The model under review builds one solid part; all positions refer to its coordinate system, in mm. Face numbers are marked on the shaded views. A direction names the side the tool comes from. Round coordinates to 2 decimals unless told otherwise and drop trailing zeros. Loops run counter-clockwise (first coordinate to the right, second up) from the corner with the lowest first, then second, coordinate; pieces in that order, holes last. Notation, with made-up numbers: M 9,-22.5 L 36,-22.5 A31 cw 36,2.5 Z; hole C 14.25,55 d9. An arc over 180 degrees is marked long. Answer in a Markdown table with one row per item. Add a question column.
from build123d import *

# Parameters (mm, degrees)
SCHIZZO1_W                   = 41
SCHIZZO1_H                   = 41
ESTRUSIONE_ESTRUSIONE1_DEPTH = 1.5
SCHIZZO5_W                   = 4.5
SCHIZZO5_H                   = 4.5
ESTRUSIONE_ESTRUSIONE2_DEPTH = 6.97
SCHIZZO6_W                   = 4.5
SCHIZZO6_H                   = 4.5
ESTRUSIONE_ESTRUSIONE3_DEPTH = 6.97
SCHIZZO7_W                   = 4.5
SCHIZZO7_H                   = 4.5
ESTRUSIONE_ESTRUSIONE4_DEPTH = 6.97
SCHIZZO8_W                   = 4.5
SCHIZZO8_H                   = 4.5
ESTRUSIONE_ESTRUSIONE5_DEPTH = 6.97
SCHIZZO9_W                   = 1
SCHIZZO9_H                   = 41
ESTRUSIONE_ESTRUSIONE6_DEPTH = 12
SCHIZZO10_W                  = 26
SCHIZZO10_H                  = 1
ESTRUSIONE_ESTRUSIONE7_DEPTH = 12
SCHIZZO11_R                  = 0.4
TAGLIO_ESTRUSIONE1_DEPTH     = 10
SCHIZZO12_R                  = 0.4
TAGLIO_ESTRUSIONE2_DEPTH     = 10


with BuildPart() as part:
    # Schizzo1 → Estrusione-Estrusione1 (new body)
    with BuildSketch(Plane.XY):
        with Locations((20.5, 20.5)):
            Rectangle(SCHIZZO1_W, SCHIZZO1_H)
    extrude(amount=ESTRUSIONE_ESTRUSIONE1_DEPTH)

    # Schizzo5 → Estrusione-Estrusione2 (add)
    with BuildSketch(Plane.XY.offset(1.5)):
        with Locations((2.25, 2.25)):
            Rectangle(SCHIZZO5_W, SCHIZZO5_H)
    extrude(amount=ESTRUSIONE_ESTRUSIONE2_DEPTH)

    # Schizzo6 → Estrusione-Estrusione3 (add)
    with BuildSketch(Plane.XY.offset(1.5)):
        with Locations((38.75, 2.25)):
            Rectangle(SCHIZZO6_W, SCHIZZO6_H)
    extrude(amount=ESTRUSIONE_ESTRUSIONE3_DEPTH)

    # Schizzo7 → Estrusione-Estrusione4 (add)
    with BuildSketch(Plane.XY.offset(1.5)):
        with Locations((2.25, 38.75)):
            Rectangle(SCHIZZO7_W, SCHIZZO7_H)
    extrude(amount=ESTRUSIONE_ESTRUSIONE4_DEPTH)

    # Schizzo8 → Estrusione-Estrusione5 (add)
    with BuildSketch(Plane.XY.offset(1.5)):
        with Locations((38.75, 38.75)):
            Rectangle(SCHIZZO8_W, SCHIZZO8_H)
    extrude(amount=ESTRUSIONE_ESTRUSIONE5_DEPTH)

    # Schizzo9 → Estrusione-Estrusione6 (add)
    with BuildSketch(Plane(origin=(0, 0, 0), x_dir=(-1, 0, 0), z_dir=(0, 0, -1))):
        with Locations((-40.5, 20.5)):
            Rectangle(SCHIZZO9_W, SCHIZZO9_H)
    extrude(amount=ESTRUSIONE_ESTRUSIONE6_DEPTH)

    # Schizzo10 → Estrusione-Estrusione7 (add)
    with BuildSketch(Plane(origin=(0, 0, 0), x_dir=(-1, 0, 0), z_dir=(0, 0, -1))):
        with Locations((-13, 40.5)):
            Rectangle(SCHIZZO10_W, SCHIZZO10_H)
    extrude(amount=ESTRUSIONE_ESTRUSIONE7_DEPTH)

    # Schizzo11 → Taglio-Estrusione1 (cut)
    with BuildSketch(Plane.XY.offset(8.47)):
        with Locations((32.781075858, 214.49933813)):
            Circle(SCHIZZO11_R)
    extrude(amount=-TAGLIO_ESTRUSIONE1_DEPTH, mode=Mode.SUBTRACT)

    # Schizzo12 → Taglio-Estrusione2 (cut)
    with BuildSketch(Plane.XY.offset(8.47)):
        with Locations((-3.518924142, 178.29933813)):
            Circle(SCHIZZO12_R)
    extrude(amount=-TAGLIO_ESTRUSIONE2_DEPTH, mode=Mode.SUBTRACT)


solid = part.part
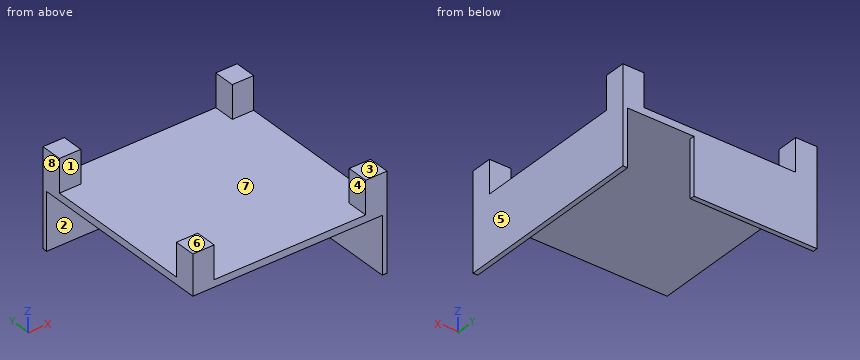
1. Take a section at A-A, the plane z = -1.75. State the section outline as (x, y) points.
2. To check wall thickness, follow probe 1 along Z at (x, y) = (20, 39.5); probe 2 along Y at (x, z) = (6, -10). State the ranges of each line that lie inside material, in increasing order.
3. For pin 1 Ø3 at (x, y) = (9.5, 26) entering from -Z; pin 2 Ø5 at (y, z) = (3.5, 6.5) entering from -X; pin 3 Ø12 at (x, y) = (19.5, 14) entering from +Z; pin 4 Ø10 at (y, z) = (31, -9) entering from -X, all flat-tipped, find the tip position at first contact; note any pin that passes through.
4. Machinability: for the marked faces 1, 2, 3 and 4, which of the approach directions +Z, -Z, +X, -X, +Y, -Y give a long, thin tool a straight path to every point of the face, cutting with its end or side? Answer none if there is none.
5. Take a section at C-C, the plane y = 13. State the section outline as (x, z) points, and give its area (3 significant figures).
6. Take a section at B-B, the plane z = 4.5. State the section outline as (x, y) points.
7. Mouldability with a two-part tool opening along X and no side actions: class the marked faces 5, 6, 7 and 8 as released by +X, released by -X, zero draft, split by the parting line, or undercut.
Check sheet entries:
| question | item | result |
|---|---|---|
| 1 | outline | M 0,40 L 26,40 L 26,41 L 0,41 Z; M 40,0 L 41,0 L 41,41 L 40,41 Z |
| 2 | probe 1 | z = 0 to 1.5 |
| 2 | probe 2 | y = 40 to 41 |
| 3 | pin 1 | stops at z = 0 |
| 3 | pin 2 | stops at x = 0 |
| 3 | pin 3 | stops at z = 1.5 |
| 3 | pin 4 | stops at x = 40 |
| 4 | face 1 | +Z, +X, -X |
| 4 | face 2 | -Z, -X, -Y |
| 4 | face 3 | +Z, +X, -X, +Y, -Y |
| 4 | face 4 | +Z, +Y, -Y |
| 5 | outline | M 0,0 L 40,0 L 40,-12 L 41,-12 L 41,1.5 L 0,1.5 Z |
| 5 | area | 73.5 mm^2 |
| 6 | outline | M 0,0 L 4.5,0 L 4.5,4.5 L 0,4.5 Z; M 0,36.5 L 4.5,36.5 L 4.5,41 L 0,41 Z; M 36.5,0 L 41,0 L 41,4.5 L 36.5,4.5 Z; M 36.5,36.5 L 41,36.5 L 41,41 L 36.5,41 Z |
| 7 | face 5 | released by +X |
| 7 | face 6 | zero draft |
| 7 | face 7 | undercut |
| 7 | face 8 | released by -X |
